```python
from build123d import *

# Parameters (mm, degrees)
F0_R     = 4.699
F1_DEPTH = 6.35


with BuildPart() as f1:
    # F0 (on Front) → F1 (new body)
    with BuildSketch(Plane.XZ):
        with BuildLine():
            ThreePointArc((-12.7, 0), (-3.719744, 3.719744), (0, 12.7))
            Line((0, 12.7), (0, 88.9))
            ThreePointArc((0, 88.9), (-0.929936, 91.145064), (-3.175, 92.075))
            Line((-3.175, 92.075), (-9.525, 92.075))
            Line((-9.525, 92.075), (-9.525, 100.33))
            ThreePointArc((-9.525, 100.33), (-9.896974, 101.228026), (-10.795, 101.6))
            Line((-10.795, 101.6), (-16.1925, 101.6))
            ThreePointArc((-16.1925, 101.6), (-17.090526, 101.228026), (-17.4625, 100.33))
            Line((-17.4625, 100.33), (-17.4625, 92.075))
            Line((-17.4625, 92.075), (-28.575, 92.075))
            ThreePointArc((-28.575, 92.075), (-44.290448, 85.565448), (-50.8, 69.85))
            Line((-50.8, 69.85), (-50.8, 3.175))
            ThreePointArc((-50.8, 3.175), (-49.870064, 0.929936), (-47.625, 0))
            Line((-47.625, 0), (-12.7, 0))
        make_face()
        with Locations((-38.1, 12.7)):
            Circle(F0_R, mode=Mode.SUBTRACT)
        with Locations((-11.1125, 69.85)):
            Circle(F0_R, mode=Mode.SUBTRACT)
    extrude(amount=F1_DEPTH)


solid = f1.part
```
Check sheet for the modelled part. Datum: model origin and axes. Units: mm. A direction names the side the tool comes from. Coordinates: 2 decimals unless noted, no trailing zeros. Order: outer loops, then holes, each group sorted by start corner. A loop starts at its lowest first (then second) coordinate and runs counter-clockwise, first axis right, second up. Notation, with made-up numbers: (-14, -29) -> (-5, -29) arc R9 ccw to (-5, -15) -> close; hole circle Ø2 at (85, -16.75). An arc over 180 degrees is marked (long way). Write each question's results on one line, items separated by ' | '. Start each with the question number.
1) Section check B-B (x = -39). Enter the section's corners in (y, z), and give its area (3 significant figures).
2) Set-up check for faces 4 (the face through (-9.525, -3, 96)), 5 (the face through (-26, -6.35, 52)), 6 (the face through (-23, -3, 92.075)): record each of +Z, -Z, +X, -X, +Y, -Y from which the full face is reachable in a straight line by a thin tool's end or side.
3) Section check C-C (z = 78). Enter the section's corners in (x, y).
4) Section check A-A (y = -2.25). Count the separate pieces of the cut face and the enclosed holes in it, and give its area (3 significant figures).
5) Section check D-D (x = -25.5). Enter the section's corners in (y, z) (3 decimals), and give its area (3 significant figures).
6) Draft check along Z on faces 1 (the face through (-13, -3, 101.6)), 2 (the face through (-8.944, -3.131, 65.681)), 3 (the face through (0, -3, 50)). Enter one of: pulls with the +Z half, pulls with the -Z half, needs draft (parallel to the pull), parting line crosses it, or undercut.
7) Material ranges on line 1 along Z through (x, y) = (-18, -2.75) (3 decimals); line 2 along Z through (x, y) = (-38, -2.5); line 3 along Z through (x, y) = (-40, -2), recorded low to high.
Checked values:
1) outline: (-6.35, 0) -> (0, 0) -> (0, 8.09) -> (-6.35, 8.09) -> close; (-6.35, 17.31) -> (0, 17.31) -> (0, 89.48) -> (-6.35, 89.48) -> close | area: 510 mm²
2) face 4: +Z, +X, +Y, -Y | face 5: +Z, -Z, +X, -X, -Y | face 6: +Z, -X, +Y, -Y
3) outline: (-49.25, -6.35) -> (0, -6.35) -> (0, 0) -> (-49.25, 0) -> close
4) separate pieces: 1 | enclosed holes: 2 | area: 4,470 mm²
5) outline: (-6.35, 0) -> (0, 0) -> (0, 92.075) -> (-6.35, 92.075) -> close | area: 585 mm²
6) face 1: pulls with the +Z half | face 2: undercut | face 3: needs draft
7) line 1: 0 to 92.075 | line 2: 0 to 8, 17.4 to 89.98 | line 3: 0 to 8.4, 17 to 88.91
